Source: CAD feature listing. Evaluate the final solid. Frame: model axes, mm. Round coordinates to 2 decimals unless told otherwise and drop trailing zeros. Order: outer loops, then holes, each group sorted by start corner. A loop starts at its lowest first (then second) coordinate and runs counter-clockwise, first axis right, second up. Notation, with made-up numbers: (37.5, -19) - (71.5, -19) arc R9 cw to (71.5, -10) - close; hole circle Ø6 at (53.5, -9). An arc over 180 degrees is marked (long way). Use one line per item in the form item = value. Start each with the question number.
Q1. Pin query (flat end, axial travel): pin 1 Ø5 at (x, y) = (-7, 3.5) entering from -Z; pin 2 Ø3 at (y, z) = (-5.5, 5.5) entering from +X; pin 3 Ø5 at (x, z) = (0.5, 4) entering from -Y; pin 4 Ø1.5 at (y, z) = (-5, 2) entering from +X. Return the tip coordinate at first contact, or that it passes through.
Q2. Draft query along X for faces 1 (the flat face through (2, -6, 1)), 2 (the cylindrical face through (-6, 0, 5)), 3 (the cylindrical face through (-1.08, -4.88, 4.44)). Return one class per face: released by +X, released by -X, zero draft, split by the parting line, or undercut.
Q3. Cut plane D-D, the plane y = 7. Return the cut outline in (x, z), and give its area (3 significant figures).
Q4. Cut plane C-C, the plane z = 2. Return the cut outline in (x, y), and give its area (3 significant figures).
Q5. Cut plane A-A, the plane x = 0. Return the cut outline in (y, z), and give its area (3 significant figures).
Q6. Ray query, line 1 (Y direction, x = 0, z = 6.25); line 2 (Z direction, x = -5, y = 7); line 3 (X direction, y = -0.75, z = 8). Return the intervals inside material, ascending. Write a range as [from, to].
from build123d import *

# Parameters (mm, degrees)
SKETCH1_R           = 9
SKETCH1_R_2         = 5
BOSS_EXTRUDE1_DEPTH = 1
SKETCH2_R           = 6
SKETCH2_R_2         = 5
BOSS_EXTRUDE2_DEPTH = 8
CHAMFER1_SIZE       = 0.3


with BuildPart() as part:
    # Sketch1 → Boss-Extrude1 (new body)
    with BuildSketch(Plane.XY):
        Circle(SKETCH1_R)
        Circle(SKETCH1_R_2, mode=Mode.SUBTRACT)
    extrude(amount=BOSS_EXTRUDE1_DEPTH)

    # Sketch2 → Boss-Extrude2 (add)
    with BuildSketch(Plane.XY.offset(1)):
        Circle(SKETCH2_R)
        Circle(SKETCH2_R_2, mode=Mode.SUBTRACT)
    extrude(amount=BOSS_EXTRUDE2_DEPTH)

    # Chamfer1
    chamfer1_edges = [part.edges().sort_by_distance(p)[0] for p in [
        (-6, 0, 9),
    ]]
    chamfer(chamfer1_edges, length=CHAMFER1_SIZE)


solid = part.part
Completed:
q1.pin_1 = 0
q1.pin_2 = 4.47
q1.pin_3 = -6
q1.pin_4 = 4.24
q2.face_1 = zero draft
q2.face_2 = split by the parting line
q2.face_3 = undercut
q3.outline = (-5.66, 0) - (5.66, 0) - (5.66, 1) - (-5.66, 1) - close
q3.area = 11.3 mm2
q4.outline = circle Ø12 at (0, 0); hole circle Ø10 at (0, 0)
q4.area = 34.6 mm2
q5.outline = (-9, 0) - (-5, 0) - (-5, 9) - (-5.7, 9) - (-6, 8.7) - (-6, 1) - (-9, 1) - close; (5, 0) - (9, 0) - (9, 1) - (6, 1) - (6, 8.7) - (5.7, 9) - (5, 9) - close
q5.area = 23.9 mm2
q6.line_1 = [-6, -5], [5, 6]
q6.line_2 = [0, 1]
q6.line_3 = [-5.95, -4.94], [4.94, 5.95]
